Geometry: final body of the model. Coordinates: model frame, mm. A direction names the side the tool comes from. Round coordinates to 2 decimals unless told otherwise and drop trailing zeros. Order: outer loops, then holes, each group sorted by start corner. A loop starts at its lowest first (then second) coordinate and runs counter-clockwise, first axis right, second up. Notation, with made-up numbers: M 48,53 L 71,53 A23 cw 71,64 Z; hole C 56,-31 d11. An arc over 180 degrees is marked long. Put each result on its own line as item: value. Start each with the question number.
1) Access query for faces 1 (the flat face through (3, -3, 0)), 2 (the conical face through (-4.745, 9.123, 4.677)). Directions: +Z, -Z, +X, -X, +Y, -Y. A direction counts if a zero-diameter tool reaches every point of the face in a straight line with its end or side. Return the directions, or none.
2) Section A-A, the plane x = 0. Return loops of the section in (y, z), then the cut area to 3 significant figures.
3) Section C-C, the plane z = 10. Return loops of the section in (x, y), then the cut area to 3 significant figures.
4) First-contact query: P1, Ø10, axis at x = 1.5, y = -1.5, coming from the -Z side; P2, Ø1, axis at y = 7, z = 4, coming from the +X side; P3, Ø5, axis at y = -1.5, z = 9, coming from the +X side; P4, Ø1, axis at y = -6, z = 15, coming from the +X side. Flat tips, straight axial feed; report the tip coordinate or a pass-through.
5) Material intervals for probe 1 along Y at (x, z) = (0, 14); probe 2 along Z at (x, y) = (0, 9); probe 3 along Y at (x, z) = (0, 29.5), sorted ascending. Write a range as [from, to].
6) Draft query along Y for faces 3 (the flat face through (-1, -8, 8.8)), 4 (the conical face through (2.237, 10.074, 33.459)), 5 (the cylindrical face through (-3.852, -1.213, 18.783)). Return one class per face: pulls with the +Y half, pulls with the -Y half, needs draft (parallel to the pull), parting line crosses it, or undercut.
from build123d import *

# Parameters (mm, degrees)
SKETCH1_R           = 12.7
SKETCH1_R_2         = 4.0386
BOSS_EXTRUDE1_DEPTH = 38.1


with BuildPart() as part:
    # Sketch1 → Boss-Extrude1 (new body)
    with BuildSketch(Plane.XY):
        with Locations(Location((0, 0, 0), (0, 0, 180))):
            Circle(SKETCH1_R)
        with Locations(Location((0, 0, 0), (0, 0, 180))):
            Circle(SKETCH1_R_2, mode=Mode.SUBTRACT)
    extrude(amount=BOSS_EXTRUDE1_DEPTH)

    # Sketch2 → Cut-Revolve1 (revolve, cut)
    with BuildSketch(Plane(origin=(0, 0, 0), x_dir=(1, 0, 0), z_dir=(0, 1, 0)), mode=Mode.PRIVATE) as cut_revolve1_sk:
        Polygon((10.16, -33.3), (12.7, -35.84), (12.7, -2.26), (10.16, -4.8), (10.16, -8.8), (7.62, -8.8), (7.62, -29.3), (10.16, -29.3), align=None)
    revolve(cut_revolve1_sk.sketch.rotate(Axis((0, 0, 0), (0, 0, 1)), 180), axis=Axis((0, 0, 0), (0, 0, 1)), mode=Mode.SUBTRACT)


solid = part.part
Result sheet:
1. face 1: -Z, +X, -X, +Y, -Y
1. face 2: none
2. outline: M -12.7,0 L -4.04,0 L -4.04,38.1 L -12.7,38.1 L -12.7,35.84 L -10.16,33.3 L -10.16,29.3 L -7.62,29.3 L -7.62,8.8 L -10.16,8.8 L -10.16,4.8 L -12.7,2.26 Z; M 4.04,0 L 12.7,0 L 12.7,2.26 L 10.16,4.8 L 10.16,8.8 L 7.62,8.8 L 7.62,29.3 L 10.16,29.3 L 10.16,33.3 L 12.7,35.84 L 12.7,38.1 L 4.04,38.1 Z
2. area: 398 mm2
3. outline: C 0,0 d15.24; hole C 0,0 d8.08
3. area: 131 mm2
4. P1: stops at z = 0
4. P2: stops at x = 9.18
4. P3: stops at x = 10.16
4. P4: stops at x = 5.27
5. probe 1: y = [-7.62, -4.04], [4.04, 7.62]
5. probe 2: z = [0, 8.8], [29.3, 38.1]
5. probe 3: y = [-10.16, -4.04], [4.04, 10.16]
6. face 3: needs draft
6. face 4: parting line crosses it
6. face 5: undercut
